from build123d import *

# Parameters (mm, degrees)
SKETCH3_R          = 2
CUT_EXTRUDE1_DEPTH = 10
SKETCH4_R          = 2
CUT_EXTRUDE2_DEPTH = 10


with BuildPart() as part:
    # Sketch1 → Revolve3 (revolve)
    with BuildSketch(Plane.XY, mode=Mode.PRIVATE) as revolve3_sk:
        with BuildLine():
            Line((-6.205707302, 80), (-24.563281142, 80))
            Line((-24.563281142, 80), (-24.563281142, 110))
            ThreePointArc((-24.563281142, 110), (-111.666310606, 82.552480161), (-178.205707302, 20))
            Line((-178.205707302, 20), (-213.033718137, 20))
            Line((-213.033718137, 20), (-239.205707302, 48.265748299))
            Line((-239.205707302, 48.265748299), (-249.205707302, 48.265748299))
            Line((-249.205707302, 48.265748299), (-249.205707302, 30))
            Line((-249.205707302, 30), (-259.205707302, 30))
            Line((-259.205707302, 30), (-259.205707302, 55))
            Line((-259.205707302, 55), (-256.705707302, 55))
            Line((-256.705707302, 55), (-256.705707302, 53))
            Line((-256.705707302, 53), (-236.705707302, 53))
            Line((-236.705707302, 53), (-236.705707302, 55))
            Line((-236.705707302, 55), (-234.205707302, 55))
            Line((-234.205707302, 55), (-209.205707302, 28))
            Line((-209.205707302, 28), (-207.31461189, 28))
            Line((-207.31461189, 28), (-207.31461189, 26))
            Line((-207.31461189, 26), (-187.31461189, 26))
            Line((-187.31461189, 26), (-187.31461189, 28))
            Line((-187.31461189, 28), (-184.205707302, 28))
            ThreePointArc((-184.205707302, 28), (-167.911507534, 48.712256642), (-149.205707302, 67.275434145))
            Line((-149.205707302, 67.275434145), (-149.205707302, 75.5))
            Line((-149.205707302, 75.5), (-129.205707302, 75.5))
            Line((-129.205707302, 75.5), (-129.205707302, 82.838508469))
            ThreePointArc((-129.205707302, 82.838508469), (-109.780198591, 94.730106924), (-89.205707302, 104.5))
            Line((-89.205707302, 104.5), (-69.205707302, 104.5))
            Line((-69.205707302, 104.5), (-69.205707302, 111.59643719))
            ThreePointArc((-69.205707302, 111.59643719), (-49.395048279, 116.53049781), (-29.205707302, 119.563264874))
            Line((-29.205707302, 119.563264874), (-29.205707302, 117.5))
            Line((-29.205707302, 117.5), (-9.205707302, 117.5))
            Line((-9.205707302, 117.5), (-9.205707302, 120))
            Line((-9.205707302, 120), (-6.205707302, 120))
            Line((-6.205707302, 120), (-6.205707302, 80))
        make_face()
    revolve(revolve3_sk.sketch.rotate(Axis((-303.234759745, 0, 0), (1, 0, 0)), 90), axis=Axis((-303.234759745, 0, 0), (1, 0, 0)))

    # Sketch3 → Cut-Extrude1 (cut)
    with BuildSketch(Plane(origin=(-6.205707302, 0, 0), x_dir=(0, 0, -1), z_dir=(1, 0, 0))):
        with Locations((0, 92)):
            Circle(SKETCH3_R)
        with Locations((54.076243211, 74.429563482)):
            Circle(SKETCH3_R)
        with Locations((87.497199499, 28.429563482)):
            Circle(SKETCH3_R)
        with Locations((87.497199499, -28.429563482)):
            Circle(SKETCH3_R)
        with Locations((54.076243211, -74.429563482)):
            Circle(SKETCH3_R)
        with Locations((0, -92)):
            Circle(SKETCH3_R)
        with Locations((-54.076243211, -74.429563482)):
            Circle(SKETCH3_R)
        with Locations((-87.497199499, -28.429563482)):
            Circle(SKETCH3_R)
        with Locations((-87.497199499, 28.429563482)):
            Circle(SKETCH3_R)
        with Locations((-54.076243211, 74.429563482)):
            Circle(SKETCH3_R)
    extrude(amount=-CUT_EXTRUDE1_DEPTH, mode=Mode.SUBTRACT)

    # Sketch4 → Cut-Extrude2 (cut)
    with BuildSketch(Plane.ZY.offset(259.205707302)):
        with Locations((0, 47.5)):
            Circle(SKETCH4_R)
        with Locations((27.919799484, 38.428307233)):
            Circle(SKETCH4_R)
        with Locations((45.175184524, 14.678307233)):
            Circle(SKETCH4_R)
        with Locations((45.175184524, -14.678307233)):
            Circle(SKETCH4_R)
        with Locations((27.919799484, -38.428307233)):
            Circle(SKETCH4_R)
        with Locations((0, -47.5)):
            Circle(SKETCH4_R)
        with Locations((-27.919799484, -38.428307233)):
            Circle(SKETCH4_R)
        with Locations((-45.175184524, -14.678307233)):
            Circle(SKETCH4_R)
        with Locations((-45.175184524, 14.678307233)):
            Circle(SKETCH4_R)
        with Locations((-27.919799484, 38.428307233)):
            Circle(SKETCH4_R)
    extrude(amount=-CUT_EXTRUDE2_DEPTH, mode=Mode.SUBTRACT)


solid = part.part
Model file for the job. Use its own axes, mm. A direction names the side the tool comes from. Give positions to 0.01 mm unless a question says otherwise; leave off trailing zeros. Loops run counter-clockwise (first coordinate to the right, second up) from the corner with the lowest first, then second, coordinate; pieces in that order, holes last. Notation, with made-up numbers: (7, 68) -> (19, 68) arc R13 cw to (19, 89) -> close; hole circle Ø9 at (15.25, 85). An arc over 180 degrees is marked (long way). Use a Markdown table: item, result. Add a question column.
(1) Slice it at B-B on x = -191.5. List the corners of the cut face in (y, z).
(2) Tool access for faces 1 (the flat face through (-236.706, -29, 45)), 2 (the cylindrical face through (-15.513, -3.517, -79.923)), 3 (the flat face through (-129.206, 36, -67)): list every direction of +Z, -Z, +X, -X, +Y, -Y with a clear straight run to the whole face (end or side of a thin tool).
(3) Wall check: line 1 along X through (y, z) = (38.5, 11); line 2 along Y through (x, z) = (-12.5, 0); line 3 along X through (y, z) = (26.5, 39). Give the ranges that are in metal, low to high.
(4) Drop flat-ended pins along their axis: pin 1 Ø2.5 at (y, z) = (28.43, 87.5) entering from +X; pin 2 Ø1.3 at (y, z) = (39.5, -28.5) entering from -X; pin 3 Ø3 at (y, z) = (-30.5, 56.5) entering from +X. Give the stop position or say it passes through.
(5) Slice it at A-A on x = -243. List the corners of the cut face in (y, z).
(6) Mould opens along Z. For faces 4 (the cylindrical face through (-246.57, -52.55, -6.9)), 5 (the flat face through (-69.206, -100, -33)), 6 (the flat face through (-24.563, 81, -8)) say: +Z half, -Z half, draft (parallel to the pull), parting line (faces both ways), or undercut.
Filled sheet:
| question | item | result |
|---|---|---|
| 1 | outline | circle Ø52 at (0, 0); hole circle Ø40 at (0, 0) |
| 2 | face 1 | none |
| 2 | face 2 | +X |
| 2 | face 3 | -X |
| 3 | line 1 | -259.21 to -249.21, -231.59 to -220.35, -175.24 to -162.87 |
| 3 | line 2 | -117.5 to -94, -90 to -80, 80 to 90, 94 to 117.5 |
| 3 | line 3 | -259.21 to -249.21, -238.17 to -226.94, -169.29 to -156.4 |
| 4 | pin 1 | x = -16.21 |
| 4 | pin 2 | x = -249.21 |
| 4 | pin 3 | x = -136.16 |
| 5 | outline | circle Ø106 at (0, 0); hole circle Ø96.53 at (0, 0) |
| 6 | face 4 | parting line |
| 6 | face 5 | draft |
| 6 | face 6 | undercut |
